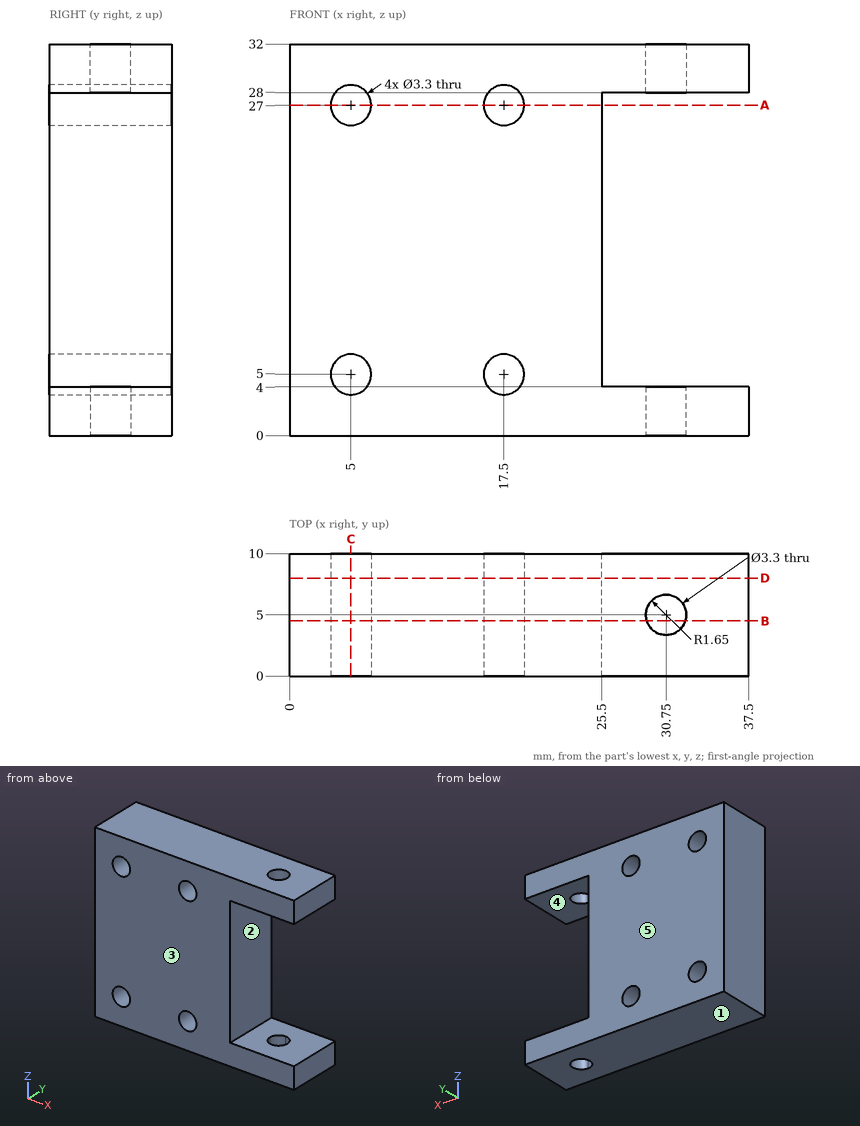
Can you work these out from the drawing? Everything is in mm from the part's minimum corner. A direction names the side the tool comes from. Round coordinates to 2 decimals unless told otherwise and drop trailing zeros. Order: outer loops, then holes, each group sorted by start corner. A loop starts at its lowest first (then second) coordinate and runs counter-clockwise, first axis right, second up.
(1) If we section it at C-C (x = 5): Please give me the cut outline in (y, z), plus the area to 3 significant figures.
Results are:
outline: (0, 0) - (10, 0) - (10, 3.35) - (0, 3.35) - close; (0, 6.65) - (10, 6.65) - (10, 25.35) - (0, 25.35) - close; (0, 28.65) - (10, 28.65) - (10, 32) - (0, 32) - close
area: 254 mm2
(2) If we section it at B-B (y = 4.5): Please give me the cut outline in (x, z).
Results are:
outline: (0, 0) - (29.18, 0) - (29.18, 4) - (25.5, 4) - (25.5, 28) - (29.18, 28) - (29.18, 32) - (0, 32) - close; (32.32, 0) - (37.5, 0) - (37.5, 4) - (32.32, 4) - close; (32.32, 28) - (37.5, 28) - (37.5, 32) - (32.32, 32) - close; hole circle Ø3.3 at (5, 5); hole circle Ø3.3 at (5, 27); hole circle Ø3.3 at (17.5, 5); hole circle Ø3.3 at (17.5, 27)
(3) I'm going to push flat-ended pins straight in: pin 1 (1 mm diameter, centred on y = 3.5, z = 23, fed in from +X); pin 2 (2 mm diameter, centred on x = 30.75, y = 5, fed in from +Z). Where does each tip first touch, or does it pass through?
Results are:
pin 1: stops at x = 25.5
pin 2: passes through
(4) We'd pull the mould along Z, two halves only. Please class the marked faces 1, 2 and 3: +Z half, -Z half, draft (parallel to the pull), parting line (faces both ways), or undercut.
Results are:
face 1: -Z half
face 2: undercut
face 3: draft
(5) If we section it at D-D (y = 8): Please give me the cut outline in (x, z).
Results are:
outline: (0, 0) - (37.5, 0) - (37.5, 4) - (25.5, 4) - (25.5, 28) - (37.5, 28) - (37.5, 32) - (0, 32) - close; hole circle Ø3.3 at (5, 5); hole circle Ø3.3 at (5, 27); hole circle Ø3.3 at (17.5, 5); hole circle Ø3.3 at (17.5, 27)
(6) If I drill on L1, parallel to X at y = 3.75, z = 27; L2, parallel to Z at x = 35, y = 4; L3, parallel to X at y = 1.5, z = 15, over which ranges is the centre line in solid material (lowest first)?
Results are:
L1: x = 0 to 3.35, 6.65 to 15.85, 19.15 to 25.5
L2: z = 0 to 4, 28 to 32
L3: x = 0 to 25.5
(7) If we section it at A-A (z = 27): Please give me the cut outline in (x, y), plus the area to 3 significant figures.
Results are:
outline: (0, 0) - (3.35, 0) - (3.35, 10) - (0, 10) - close; (6.65, 0) - (15.85, 0) - (15.85, 10) - (6.65, 10) - close; (19.15, 0) - (25.5, 0) - (25.5, 10) - (19.15, 10) - close
area: 189 mm2
(8) On a 3-axis mill with a long thin cutter (end or side, diameter ignored), from which of +Z, -Z, +X, -X, +Y, -Y can I reach the whole of each face in a straight line? I mean the marked faces 4 and 5. Say none if no direction works.
Results are:
face 4: +X, +Y, -Y
face 5: +Z, -Z, +X, -X, +Y
